Autodesk Inventor part; units mm, degrees
ref_plane "YZ Plane" through (0, 0, 0) normal (1, 0, 0) x (0, 1, 0)
ref_plane "XZ Plane" through (0, 0, 0) normal (0, 1, 0) x (-1, 0, 0)
ref_plane "XY Plane" through (0, 0, 0) normal (0, 0, 1) x (1, 0, 0)
sketch "スケッチ1" plane through (0, 0, 0) normal (0, 0, 1) x (1, 0, 0)
  circle A0 centre (0, 0) radius 3.25
  circle A1 centre (0, 0) radius 2
  line L0 (0, -4.0415) -> (-3.5, -2.0207)
  line L1 (-3.5, -2.0207) -> (-3.5, 2.0207)
  line L2 (-3.5, 2.0207) -> (0, 4.0415)
  line L3 (0, 4.0415) -> (3.5, 2.0207)
  line L4 (3.5, 2.0207) -> (3.5, -2.0207)
  line L5 (3.5, -2.0207) -> (0, -4.0415)
  dimension "d0" = 6.5
  dimension "d1" = 4
  dimension "d2" = 7
extrude "押し出し1" add sketch "スケッチ1" along normal blind 1.9 contours A0
extrude "押し出し2" add sketch "スケッチ1" along normal blind 0.6 contours L0 L1 L2 L3 L4 L5
thread "ねじ1"
properties part number "SF419" material "チタン"
The listing builds one solid part. Answer for the finished solid, in the listing's coordinates (mm). A direction names the side the tool comes from. Give positions to 0.01 mm unless a question says otherwise; leave off trailing zeros. Order: outer loops, then holes, each group sorted by start corner. A loop starts at its lowest first (then second) coordinate and runs counter-clockwise, first axis right, second up. Notation, with made-up numbers: M -33,74.5 L 19,74.5 A20 cw 19,88.5 Z; hole C -1.5,18 d7. An arc over 180 degrees is marked long. Put each result on its own line as item: value. Start each with the question number.
Item 1: Find the intervals of material crossed by line 1 along Y through (x, z) = (0, 0.95); line 2 along Z through (x, y) = (3, -2.25); line 3 along X through (y, z) = (-0.5, 1.2), in increasing order.
Item 2: The part is cut by section D-D, the plane x = -3. Determine the outline of the cut face in (y, z), and give its area (3 significant figures).
Item 3: The part is cut by section C-C, the plane x = 1.5. Determine the outline of the cut face in (y, z), and give its area (3 significant figures).
Item 4: Which of the six approach directions +Z, -Z, +X, -X, +Y, -Y give full straight-line access (tool end or side, diameter ignored) to faces 1 (the face through (-2.579, 1.978, 1.241)), 2 (the face through (1.726, 3.045, 0.296))?
Item 5: The part is cut by section B-B, the plane z = 0.3. Determine the outline of the cut face in (x, y).
Item 6: For a pull along X with two mould halves and no side action, classify faces 3 (the face through (0, 2, 1)), 4 (the face through (-1.8, 3, 0.3)), 5 (the face through (1.8, -3, 0.3)) as +X half, -X half, draft (parallel to the pull), parting line (faces both ways), or undercut.
Item 7: The part is cut by section A-A, the plane y = 0. Determine the outline of the cut face in (x, z).
Answer key:
1. line 1: y = -3.25 to -2, 2 to 3.25
1. line 2: z = 0 to 0.6
1. line 3: x = -3.21 to -1.94, 1.94 to 3.21
2. outline: M -2.31,0 L 2.31,0 L 2.31,0.6 L 1.25,0.6 L 1.25,1.9 L -1.25,1.9 L -1.25,0.6 L -2.31,0.6 Z
2. area: 6.02 mm²
3. outline: M -3.18,0 L -1.32,0 L -1.32,1.9 L -2.88,1.9 L -2.88,0.6 L -3.18,0.6 Z; M 1.32,0 L 3.18,0 L 3.18,0.6 L 2.88,0.6 L 2.88,1.9 L 1.32,1.9 Z
3. area: 6.28 mm²
4. face 1: +Z
4. face 2: +Z, -Z, +X, +Y
5. outline: M -3.5,-2.02 L 0,-4.04 L 3.5,-2.02 L 3.5,2.02 L 0,4.04 L -3.5,2.02 Z; hole C 0,0 d4
6. face 3: undercut
6. face 4: -X half
6. face 5: +X half
7. outline: M -3.5,0 L -2,0 L -2,1.9 L -3.25,1.9 L -3.25,0.6 L -3.5,0.6 Z; M 2,0 L 3.5,0 L 3.5,0.6 L 3.25,0.6 L 3.25,1.9 L 2,1.9 Z
